```python
from build123d import *

# Parameters (mm, degrees)
F0_W           = 85
F0_H           = 47
F1_DEPTH       = 19
F3_DEPTH       = 85.001
F4_R           = 3.3
F5_DEPTH       = 38.001
F7_D           = 4.3
F7_CSINK_D     = 9
F7_CSINK_ANGLE = 90
F8_R           = 10


with BuildPart() as f1:
    # F0 (on Front) → F1 (new body, symmetric)
    with BuildSketch(Plane.XZ):
        Rectangle(F0_W, F0_H)
    extrude(amount=F1_DEPTH, both=True)

    # F2 (on face) → F3 (cut, through all)
    with BuildSketch(Plane(origin=(-42.5, 0, 0), x_dir=(0, -1, 0), z_dir=(-1, 0, 0))):
        with BuildLine():
            Line((-14.35, 3.5), (-14.35, -18.5))
            Line((-14.35, -18.5), (14.35, -18.5))
            Line((14.35, -18.5), (14.35, 3.5))
            ThreePointArc((14.35, 3.5), (9, 12.93808773), (14.35, 22.3761754601))
            Line((14.35, 22.3761754601), (14.35, 23.5))
            Line((14.35, 23.5), (-14.35, 23.5))
            Line((-14.35, 23.5), (-14.35, 22.3761754601))
            ThreePointArc((-14.35, 22.3761754601), (-9, 12.93808773), (-14.35, 3.5))
        make_face()
    extrude(amount=-F3_DEPTH, mode=Mode.SUBTRACT)

    # F4 (on face) → F5 (cut, through all)
    with BuildSketch(Plane.XZ.offset(19)):
        with Locations((12.5, 12.93808773)):
            Circle(F4_R)
    extrude(amount=-F5_DEPTH, mode=Mode.SUBTRACT)

    # F7 (through all)
    with Locations(Plane.XY.offset(-18.5)):
        with Locations((-30.5, 0), (30.5, 0)):
            CounterSinkHole(F7_D / 2, F7_CSINK_D / 2, counter_sink_angle=F7_CSINK_ANGLE)

    # F8
    f8_edges = [f1.edges().sort_by_distance(p)[0] for p in [
        (-42.5, 16.675, 23.5),
        (-42.5, -16.675, 23.5),
        (42.5, 16.675, 23.5),
        (42.5, -16.675, 23.5),
    ]]
    fillet(f8_edges, radius=F8_R)


solid = f1.part
```
Part model, mm, in its own coordinate system. A direction names the side the tool comes from. Round coordinates to 2 decimals unless told otherwise and drop trailing zeros. Loops run counter-clockwise (first coordinate to the right, second up) from the corner with the lowest first, then second, coordinate; pieces in that order, holes last. Notation, with made-up numbers: (-25.5, 53) -> (28.5, 53) arc R27 ccw to (28.5, 79) -> close; hole circle Ø2 at (25, 11.25). An arc over 180 degrees is marked (long way). Use one line per item in the form item = value. Start each with the question number.
Item 1: Band-saw the part on C-C (y = -11.5). List the corners of the cut face in (x, z).
Item 2: Drill centre lines: line 1 along X through (y, z) = (0, -21.95); line 2 along Y through (x, z) = (-14.5, -2). Where is each one in solid material? Low to high.
Item 3: Band-saw the part on D-D (x = 11.5). List the corners of the cut face in (y, z), plus the area to 3 significant figures.
Item 4: Band-saw the part on A-A (z = 2). List the corners of the cut face in (x, y), plus the area to 4 significant figures.
Item 5: Drop flat-ended pins along their axis: pin 1 Ø5.5 at (x, y) = (-30.5, 0) entering from -Z; pin 2 Ø5 at (x, y) = (-10, -8.5) entering from +Z; pin 3 Ø6 at (y, z) = (13, 18) entering from -X; pin 4 Ø1.5 at (x, y) = (28, -2) entering from +Z. Give the stop position or say it passes through.
Item 6: Band-saw the part on B-B (x = -30.5). List the corners of the cut face in (y, z), plus the area to 3 significant figures.
Item 7: Tool access for faces 5 (the cylindrical face through (-1, 9, 13)), 6 (the flat face through (42.5, 1, -19)): list every direction of +Z, -Z, +X, -X, +Y, -Y with a clear straight run to the whole face (end or side of a thin tool).
Item 8: Two-plate mould, pull along Z, no slides. Class faces 1 (the flat face through (-1, 19, 0)), 2 (the flat face through (-1, 14.35, -7)), 3 (the flat face through (-1, -14.35, -8)), 4 (the conical face through (-32.66, 0.68, -20.736)): released by +Z, released by -Z, zero draft, split by the parting line, or undercut.
Data:
q1.outline = (-42.5, -23.5) -> (42.5, -23.5) -> (42.5, -18.5) -> (-42.5, -18.5) -> close; (-42.5, 5.96) -> (42.5, 5.96) -> (42.5, 13.5) arc R10 ccw to (40.17, 19.92) -> (-40.17, 19.92) arc R10 ccw to (-42.5, 13.5) -> close; hole circle Ø6.6 at (12.5, 12.94)
q2.line_1 = -42.5 to -32.65, -28.35 to 28.35, 32.65 to 42.5
q2.line_2 = -19 to -14.35, 14.35 to 19
q3.outline = (-19, -23.5) -> (19, -23.5) -> (19, 9.79) -> (9.46, 9.79) arc R11 ccw to (14.35, 3.5) -> (14.35, -18.5) -> (-14.35, -18.5) -> (-14.35, 3.5) arc R11 ccw to (-9.46, 9.79) -> (-19, 9.79) -> close; (-19, 16.08) -> (-9.46, 16.08) arc R11 ccw to (-14.35, 22.38) -> (-14.35, 23.5) -> (-19, 23.5) -> close; (9.46, 16.08) -> (19, 16.08) -> (19, 23.5) -> (14.35, 23.5) -> (14.35, 22.38) arc R11 ccw to start
q3.area = 600 mm^2
q4.outline = (-42.5, -19) -> (42.5, -19) -> (42.5, -14.35) -> (-42.5, -14.35) -> close; (-42.5, 14.35) -> (42.5, 14.35) -> (42.5, 19) -> (-42.5, 19) -> close
q4.area = 790.5 mm^2
q5.pin_1 = -23.5
q5.pin_2 = 19.26
q5.pin_3 = -42.39
q5.pin_4 = -19.05
q6.outline = (-19, -23.5) -> (-2.15, -23.5) -> (-2.15, -20.85) -> (-4.5, -18.5) -> (-14.35, -18.5) -> (-14.35, 3.5) arc R11 ccw to (-14.35, 22.38) -> (-14.35, 23.5) -> (-19, 23.5) -> close; (2.15, -23.5) -> (19, -23.5) -> (19, 23.5) -> (14.35, 23.5) -> (14.35, 22.38) arc R11 ccw to (14.35, 3.5) -> (14.35, -18.5) -> (4.5, -18.5) -> (2.15, -20.85) -> close
q6.area = 697 mm^2
q7.face_5 = +X, -X
q7.face_6 = +Z, -Z, +X, +Y, -Y
q8.face_1 = zero draft
q8.face_2 = undercut
q8.face_3 = undercut
q8.face_4 = released by +Z
